Build history of the part. All positions in model axes, mm. A direction names the side the tool comes from. Coordinates: 2 decimals unless noted, no trailing zeros. Write each loop counter-clockwise with the first axis right and the second up, starting at its lowest first coordinate (ties: lowest second). Pieces come first, ordered by that corner, then holes.
```python
from build123d import *

# Parameters (mm, degrees)
SKETCH1_W           = 46
SKETCH1_H           = 15
BOSS_EXTRUDE1_DEPTH = 3
SKETCH3_W           = 2.5
SKETCH3_H           = 15
BOSS_EXTRUDE2_DEPTH = 20
SKETCH4_W           = 20
SKETCH4_H           = 3
BOSS_EXTRUDE3_DEPTH = 7
SKETCH5_R           = 2
CUT_EXTRUDE1_DEPTH  = 7
SKETCH7_W           = 9.5
SKETCH7_H           = 15
BOSS_EXTRUDE4_DEPTH = 10
SKETCH8_R           = 2
CUT_EXTRUDE2_DEPTH  = 10
CUT_EXTRUDE3_DEPTH  = 43.5


with BuildPart() as part:
    # Sketch1 → Boss-Extrude1 (new body)
    with BuildSketch(Plane.XY):
        with Locations((23, 7.5)):
            Rectangle(SKETCH1_W, SKETCH1_H)
    extrude(amount=BOSS_EXTRUDE1_DEPTH)

    # Sketch3 → Boss-Extrude2 (add)
    with BuildSketch(Plane.XY.offset(3)):
        with Locations((1.25, 7.5)):
            Rectangle(SKETCH3_W, SKETCH3_H)
    boss_extrude2 = extrude(amount=BOSS_EXTRUDE2_DEPTH)

    # Sketch4 → Boss-Extrude3 (add)
    with BuildSketch(Plane.ZY):
        with Locations((13, 13.5)):
            Rectangle(SKETCH4_W, SKETCH4_H)
    boss_extrude3 = extrude(amount=BOSS_EXTRUDE3_DEPTH)

    # Sketch5 → Cut-Extrude1 (cut)
    with BuildSketch(Plane(origin=(0, 15, 0), x_dir=(1, 0, 0), z_dir=(0, 1, 0))):
        with Locations(Location((-2.25, -18.1, 0), (0, 0, 270))):
            Circle(SKETCH5_R)
        with Locations(Location((-2.25, -7.9, 0), (0, 0, 270))):
            Circle(SKETCH5_R)
    cut_extrude1 = extrude(amount=-CUT_EXTRUDE1_DEPTH, mode=Mode.SUBTRACT)

    # Mirror1: Boss-Extrude2, Boss-Extrude3, Cut-Extrude1 across plane
    add(boss_extrude2.mirror(Plane(origin=(23, 0, 0), x_dir=(0, 0, 1), z_dir=(1, 0, 0))))
    add(boss_extrude3.mirror(Plane(origin=(23, 0, 0), x_dir=(0, 0, 1), z_dir=(1, 0, 0))))
    add(cut_extrude1.mirror(Plane(origin=(23, 0, 0), x_dir=(0, 0, 1), z_dir=(1, 0, 0))), mode=Mode.SUBTRACT)

    # Sketch7 → Boss-Extrude4 (add)
    with BuildSketch(Plane.XY.offset(23)):
        with Locations((-2.25, 7.5)):
            Rectangle(SKETCH7_W, SKETCH7_H)
    boss_extrude4 = extrude(amount=BOSS_EXTRUDE4_DEPTH)

    # Sketch8 → Cut-Extrude2 (cut)
    with BuildSketch(Plane.ZY.offset(7)):
        with Locations((28, 11.25)):
            Circle(SKETCH8_R)
        with Locations((28, 3.75)):
            Circle(SKETCH8_R)
    cut_extrude2 = extrude(amount=-CUT_EXTRUDE2_DEPTH, mode=Mode.SUBTRACT)

    # Mirror4: Boss-Extrude4, Cut-Extrude2 across plane
    add(boss_extrude4.mirror(Plane.XY.offset(13)))
    add(cut_extrude2.mirror(Plane.XY.offset(13)), mode=Mode.SUBTRACT)

    # Sketch9 → Cut-Extrude3 (cut)
    with BuildSketch(Plane(origin=(2.5, 0, 0), x_dir=(0, 0, -1), z_dir=(1, 0, 0))):
        with BuildLine():
            ThreePointArc((0.608058909, 7.5), (2, -0.25), (3.391941091, 7.5))
            ThreePointArc((3.391941091, 7.5), (2, 15.25), (0.608058909, 7.5))
        make_face()
    extrude(amount=CUT_EXTRUDE3_DEPTH, mode=Mode.SUBTRACT)


solid = part.part
```
1. 3-axis set-ups, long thin cutter, end or side, ignore diameter. For faces 4 (the face through (49, 13, 3)), 5 (the face through (43.5, 7, 13)), 6 (the face through (45, 11, 23)): which of +Z, -Z, +X, -X, +Y, -Y reach the whole face in a straight line?
Computed values:
face 4: -Z, +X, +Y, -Y
face 5: +Z, +Y, -Y
face 6: +Z, +X, +Y, -Y
2. Flat gauge pins, fed straight in: pin 1 (6 mm diameter, centred on y = 9.5, z = 25.5, fed in from +X); pin 2 (4.5 mm diameter, centred on y = 5.5, z = 25.5, fed in from +X); pin 3 (1.5 mm diameter, centred on x = 3.5, y = 5, fed in from +Z); pin 4 (6.5 mm diameter, centred on x = 48.25, z = 18.1, fed in from -Y). Where does each tip first touch, or does it go through?
Computed values:
pin 1: stops at x = 46
pin 2: stops at x = 2.5
pin 3: stops at z = 3
pin 4: stops at y = 0
3. Probe line 1 along Z through (x, y) = (48.25, 13.5); line 2 along X through (y, z) = (13.8, 7.9); line 3 along Y through (x, z) = (-1, -2). List the from-to ranges inside material, lowest first.
Computed values:
line 1: z = 3 to 5.9, 9.9 to 16.1, 20.1 to 23
line 2: x = -7 to -4.25, -0.25 to 2.5, 43.5 to 46.25, 50.25 to 53
line 3: y = 0 to 1.75, 5.75 to 9.25, 13.25 to 15
4. Saw through at B-B on z = 15.5. List the corners of the cut face in (x, y), plus the area to 3 significant figures.
Computed values:
outline: (-7, 12) - (0, 12) - (0, 0) - (2.5, 0) - (2.5, 15) - (-7, 15) - close; (43.5, 0) - (46, 0) - (46, 12) - (53, 12) - (53, 15) - (43.5, 15) - close
area: 117 mm2
5. Saw through at A-A on x = -2.25. List the corners of the cut face in (y, z).
Computed values:
outline: (0, -7) - (15, -7) - (15, 5.9) - (12, 5.9) - (12, 3) - (0, 3) - close; (0, 23) - (12, 23) - (12, 20.1) - (15, 20.1) - (15, 33) - (0, 33) - close; (12, 9.9) - (15, 9.9) - (15, 16.1) - (12, 16.1) - close; hole circle Ø4 at (3.75, -2); hole circle Ø4 at (3.75, 28); hole circle Ø4 at (11.25, -2); hole circle Ø4 at (11.25, 28)
6. Saw through at D-D on x = 48.25. List the corners of the cut face in (y, z), plus the area to 3 significant figures.
Computed values:
outline: (12, 3) - (15, 3) - (15, 5.9) - (12, 5.9) - close; (12, 9.9) - (15, 9.9) - (15, 16.1) - (12, 16.1) - close; (12, 20.1) - (15, 20.1) - (15, 23) - (12, 23) - close
area: 36.0 mm2
7. Saw through at C-C on y = 3.75. List the corners of the cut face in (x, z), plus the area to 4 significant figures.
Computed values:
outline: (-7, -7) - (2.5, -7) - (2.5, -4) - (-7, -4) - close; (-7, 0) - (2.5, 0) - (2.5, 2) - (46, 2) - (46, 23) - (43.5, 23) - (43.5, 3) - (2.5, 3) - (2.5, 26) - (-7, 26) - (-7, 23) - (0, 23) - (0, 3) - (-7, 3) - close; (-7, 30) - (2.5, 30) - (2.5, 33) - (-7, 33) - close
area: 257.5 mm2
8. Mould opens along Y. For faces 1 (the face through (16.2, 15, 2.7)), 2 (the face through (2.5, 7, -2)), 3 (the face through (53, 14, 13)) say: +Y half, -Y half, draft (parallel to the pull), parting line (faces both ways), or undercut.
Computed values:
face 1: +Y half
face 2: undercut
face 3: draft
